Geometry check sheet. Reference: the model listing, model coordinates, mm. Face numbers are marked on the shaded views. A direction names the side the tool comes from. Coordinates: 2 decimals unless noted, no trailing zeros. Loops run counter-clockwise (first coordinate to the right, second up) from the corner with the lowest first, then second, coordinate; pieces in that order, holes last. Notation, with made-up numbers: (35.5, -4) - (78.5, -4) arc R34 cw to (78.5, 27) - close; hole circle Ø3 at (-28, -32). An arc over 180 degrees is marked (long way). One line per item, written item: value.
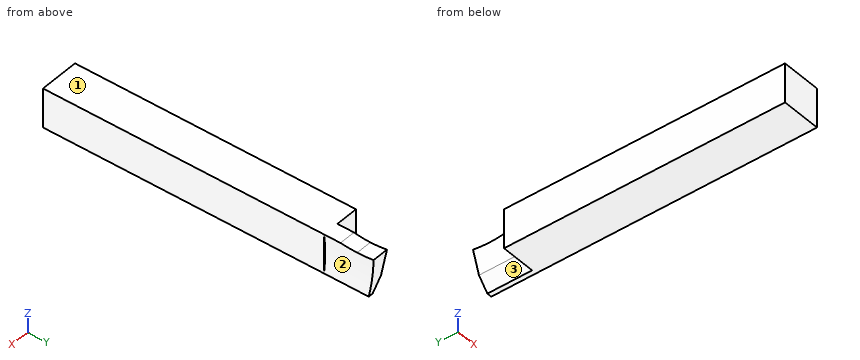
from build123d import *

# Parameters (mm, degrees)
F1_DEPTH = 12
F2_W     = 9.525
F2_H     = 9.525
F3_DEPTH = 68
F5_DEPTH = 57.25
F7_DEPTH = 57.25


with BuildPart() as f1:
    # F0 (on Front) → F1 (new body)
    with BuildSketch(Plane.XZ):
        with BuildLine():
            Line((-52.25, 0), (-56.25, 0))
            Line((-56.25, 0), (-55.3939646182, -6.0910082371))
            Line((-55.3939646182, -6.0910082371), (-53.4113485495, -9.525))
            Line((-53.4113485495, -9.525), (-52.25, -9.525))
            ThreePointArc((-52.25, -9.525), (-52.6092196059, -4.7625), (-52.25, 0))
        make_face()
    extrude(amount=F1_DEPTH)

    # F2 (on face) → F3 (join)
    with BuildSketch(Plane.XZ.offset(12)):
        with Locations((-57.0125, -4.7625)):
            Rectangle(F2_W, F2_H)
    extrude(amount=F3_DEPTH)

    # F4 (on Right) → F5 (cut, up to face)
    with BuildSketch(Plane.YZ):
        Polygon((0, -9.525), (0, 0), (-1.1695229426, -9.525), align=None)
    extrude(amount=-F5_DEPTH, mode=Mode.SUBTRACT)

    # F6 (on Right) → F7 (cut, up to face)
    with BuildSketch(Plane.YZ):
        with BuildLine():
            Line((-4, 0), (-8, 0))
            ThreePointArc((-8, 0), (-6.005617112, -0.2248948268), (-4, -0.3))
            Line((-4, -0.3), (-4, 0))
        make_face()
        with BuildLine():
            Line((0, 0), (-4, 0))
            Line((-4, 0), (-4, -0.3))
            ThreePointArc((-4, -0.3), (-1.994382888, -0.2248948268), (0, 0))
        make_face()
    extrude(amount=-F7_DEPTH, mode=Mode.SUBTRACT)


solid = f1.part
(1) Cross-section at B-B on x = -60.25. Record the cut outline in (y, z) (3 decimals).
Reply:
outline: (-80, -9.525) - (-12, -9.525) - (-12, 0) - (-80, 0) - close
(2) Material ranges on probe 1 along Y at (x, z) = (-53.75, -6); probe 2 along Y at (x, z) = (-55.75, -8.5); probe 3 along X at (y, z) = (-4, -3.25), recorded low to high. Write a range as from..to.
Reply:
probe 1: -80..-0.74
probe 2: -80..-12
probe 3: -55.79..-52.57
(3) Access from +Z, -Z, +X, -X, +Y, -Y to the whole of each face (thin tool, end or side, straight path). Record for the marked faces 1, 2 and 3.
Reply:
face 1: +Z, +X, -X, +Y, -Y
face 2: +X, +Y
face 3: -Z, -X, +Y
(4) Cross-section at C-C on x = -54.5. Record the cut outline in (y, z) (3 decimals), and give its area (3 significant figures).
Reply:
outline: (-80, -9.525) - (-12, -9.525) - (-12, -7.639) - (-0.938, -7.639) - (0, 0) arc R26.817 cw to (-8, 0) - (-80, 0) - close
area: 734 mm2
(5) Cross-section at A-A on z = -8. Record the cut outline in (x, y) (3 decimals).
Reply:
outline: (-61.775, -80) - (-52.25, -80) - (-52.25, -12) - (-52.444, -12) - (-52.444, -0.982) - (-54.292, -0.982) - (-54.292, -12) - (-61.775, -12) - close
(6) Go/stop test with a flat-tipped pin: pin 1 Ø2.5 at (x, z) = (-56, -2.5) entering from +Y. Record where the tip stops, or that it passes through.
Reply:
pin 1: y = -0.15
